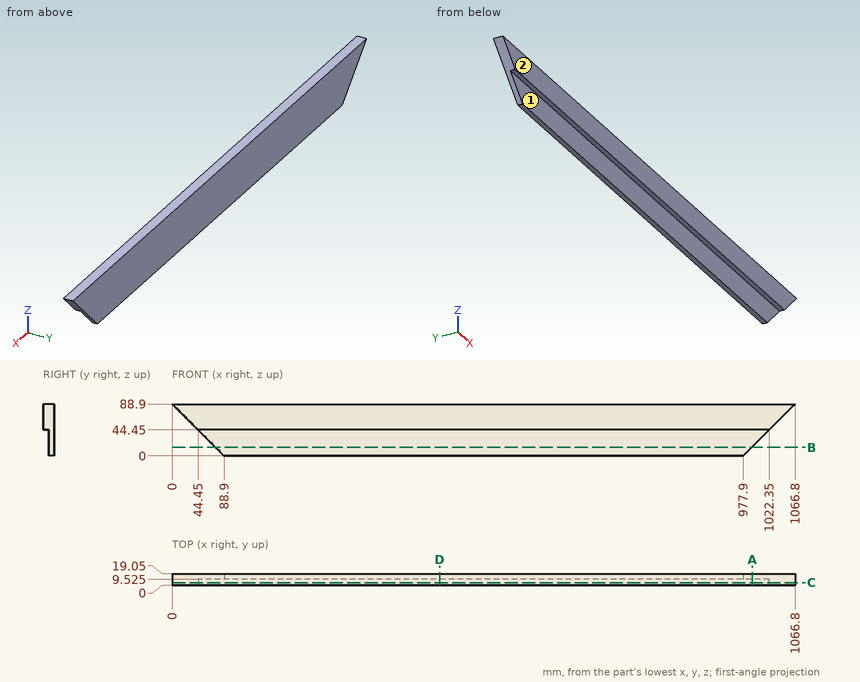
Part print with two shaded views. Sizes in mm from the minimum x, y, z corner. A direction names the side the tool comes from. Round coordinates to 2 decimals unless told otherwise and drop trailing zeros. Write each loop counter-clockwise with the first axis right and the second up, starting at its lowest first coordinate (ties: lowest second). Pieces come first, ordered by that corner, then holes. Notation, with made-up numbers: M 75.5,-40 L 133.5,-40 A28 cw 133.5,-20 Z; hole C 48.5,81 d9. An arc over 180 degrees is marked long. Answer as CSV lines item,"result". Start each with the question number.
1) Band-saw the part on A-A (x = 994). List the corners of the cut face in (y, z) (3 decimals), then the cut area to 3 significant figures.
2) Band-saw the part on B-B (z = 14.5). List the corners of the cut face in (x, y) (3 decimals).
3) Which spindle directions (+Z, -Z, +X, -X, +Y, -Y) get a long thin tool onto all of the face, cutting with end or side? Do the marked faces 1 and 2. Say none if no direction does.
4) Band-saw the part on D-D (x = 458). List the corners of the cut face in (y, z) (3 decimals), then the cut area to 3 significant figures.
5) Drill centre lines: L1, parallel to Y at x = 594.5, z = 41.5 (3 decimals); L2, parallel to Z at x = 739, y = 6; L3, parallel to X at y = 9.75, z = 34. Where is each one in solid material? Low to high.
6) Drop flat-ended pins along their axis: pin 1 (3 mm diameter, centred on y = 9, z = 78.5, fed in from -X); pin 2 (5 mm diameter, centred on x = 908.5, y = 5, fed in from -Z); pin 3 (4 mm diameter, centred on x = 565, z = 72.5, fed in from -Y); pin 4 (10 mm diameter, centred on y = 11, z = 44.5, fed in from -X). Give the stop position or say it passes through.
7) Band-saw the part on C-C (y = 4.25). List the corners of the cut face in (x, z), then the cut area to 3 significant figures.
Worked out:
1,outline,"M 0,44.45 L 9.525,44.45 L 9.525,16.1 L 19.05,16.1 L 19.05,88.9 L 0,88.9 Z"
1,area,"1,120 mm²"
2,outline,"M 74.4,9.525 L 992.4,9.525 L 992.4,19.05 L 74.4,19.05 Z"
3,face 1,"-Z, +X, -X, -Y"
3,face 2,"+Z, -Z, +X, -X, -Y"
4,outline,"M 0,44.45 L 9.525,44.45 L 9.525,0 L 19.05,0 L 19.05,88.9 L 0,88.9 Z"
4,area,"1,270 mm²"
5,L1,"9.525 to 19.05"
5,L2,"44.45 to 88.9"
5,L3,"54.9 to 1011.9"
6,pin 1,"x = 8.9"
6,pin 2,"z = 44.45"
6,pin 3,"y = 0"
6,pin 4,"x = 39.4"
7,outline,"M 0,88.9 L 44.45,44.45 L 1022.35,44.45 L 1066.8,88.9 Z"
7,area,"45,400 mm²"
